Part model, mm, in its own coordinate system. A direction names the side the tool comes from. Give positions to 0.01 mm unless a question says otherwise; leave off trailing zeros. Write each loop counter-clockwise with the first axis right and the second up, starting at its lowest first coordinate (ties: lowest second). Pieces come first, ordered by that corner, then holes. Notation, with made-up numbers: M 81.5,16 L 87.5,16 A8 cw 87.5,26 Z; hole C 19.5,46.5 d1. An arc over 180 degrees is marked long. Answer as CSV lines item,"result". Start each with the question number.
Item 1: Band-saw the part on A-A, the plane z = 2.25. List the corners of the cut face in (x, y).
Item 2: 3-axis set-ups, long thin cutter, end or side, ignore diameter. For faces 4 (the cylindrical face through (0.27, 17.78, -1.4)), 5 (the flat face through (-8, 12, -2.7)), 6 (the flat face through (10.85, 12, 4)): which of +Z, -Z, +X, -X, +Y, -Y reach the whole face in a straight line?
Item 3: Band-saw the part on B-B, the plane x = 0. List the corners of the cut face in (y, z) (3 decimals).
Item 4: Band-saw the part on C-C, the plane z = -4.5. List the corners of the cut face in (x, y) (3 decimals), then the cut area to 3 significant figures.
Item 5: Wall check: L1, parallel to Y at x = 0, z = -2; L2, parallel to X at y = 4.25, z = -2.25 (1 decimal); L3, parallel to X at y = 18.25, z = -7 (3 decimals). Give the ranges that are in metal, low to high. Write a range as from..to.
Item 6: Pin check, flat tips, straight feed: pin 1 (0.6 mm diameter, centred on x = 10, y = 13, fed in from -Z); pin 2 (1 mm diameter, centred on x = 2, y = 18, fed in from +Z); pin 3 (1.8 mm diameter, centred on x = 4.5, y = 8, fed in from -Z); pin 4 (2 mm diameter, centred on x = 0, y = 19, fed in from +Z). Stop position of each tip, or through.
Item 7: Two-plate mould, pull along X, no slides. Class faces 1 (the flat face through (9.638, 12, -2)), 2 (the flat face through (-11.5, 12, -1)), 3 (the flat face through (11.5, 12, -1)): +X half, -X half, draft (parallel to the pull), parting line (faces both ways), or undercut.
from build123d import *

# Parameters (mm, degrees)
BOSS_EXTRUDE1_DEPTH         = 25
M3_TAPPED_HOLE1_D           = 2.5
M3_TAPPED_HOLE1_CSINK_D     = 3.05
M3_TAPPED_HOLE1_CSINK_ANGLE = 90


with BuildPart() as part:
    # Sketch1 → Boss-Extrude1 (new body)
    with BuildSketch(Plane(origin=(0, 0, 0), x_dir=(1, 0, 0), z_dir=(0, 1, 0))):
        with BuildLine():
            Line((-11.5, 8.7), (-10.85, 8.7))
            Line((-10.85, 8.7), (-10.85, 2.7))
            Line((-10.85, 2.7), (-9.6375, 2.7))
            Line((-9.6375, 2.7), (-9.6375, 1.775))
            ThreePointArc((-9.6375, 1.775), (-9.0125, 1.15), (-8.3875, 1.775))
            Line((-8.3875, 1.775), (-8.3875, 2.7))
            Line((-8.3875, 2.7), (-7.175, 2.7))
            Line((-7.175, 2.7), (-7.175, 8.7))
            Line((-7.175, 8.7), (-6.675, 8.7))
            Line((-6.675, 8.7), (-6.675, 1))
            Line((-6.675, 1), (-3, 1))
            Line((-3, 1), (-3, 8.7))
            Line((-3, 8.7), (-2.5, 8.7))
            Line((-2.5, 8.7), (-2.5, 2.5))
            Line((-2.5, 2.5), (2.5, 2.5))
            Line((2.5, 2.5), (2.5, 8.7))
            Line((2.5, 8.7), (3, 8.7))
            Line((3, 8.7), (3, 1))
            Line((3, 1), (6.675, 1))
            Line((6.675, 1), (6.675, 8.7))
            Line((6.675, 8.7), (7.175, 8.7))
            Line((7.175, 8.7), (7.175, 2.7))
            Line((7.175, 2.7), (8.3875, 2.7))
            Line((8.3875, 2.7), (8.3875, 1.775))
            ThreePointArc((8.3875, 1.775), (9.0125, 1.15), (9.6375, 1.775))
            Line((9.6375, 1.775), (9.6375, 2.7))
            Line((9.6375, 2.7), (10.85, 2.7))
            Line((10.85, 2.7), (10.85, 8.7))
            Line((10.85, 8.7), (11.5, 8.7))
            Line((11.5, 8.7), (11.5, -7))
            Line((11.5, -7), (10.85, -7))
            Line((10.85, -7), (10.85, 0))
            Line((10.85, 0), (-10.85, 0))
            Line((-10.85, 0), (-10.85, -7))
            Line((-10.85, -7), (-11.5, -7))
            Line((-11.5, -7), (-11.5, 8.7))
        make_face()
    extrude(amount=BOSS_EXTRUDE1_DEPTH)

    # M3 Tapped Hole1 (through all)
    with Locations(Plane.XY):
        with Locations((0, 19)):
            CounterSinkHole(M3_TAPPED_HOLE1_D / 2, M3_TAPPED_HOLE1_CSINK_D / 2, counter_sink_angle=M3_TAPPED_HOLE1_CSINK_ANGLE)


solid = part.part
Output:
1,outline,"M -11.5,0 L -10.85,0 L -10.85,25 L -11.5,25 Z; M 10.85,0 L 11.5,0 L 11.5,25 L 10.85,25 Z"
2,face 4,"+Z, -Z"
2,face 5,"-Z, +Y, -Y"
2,face 6,"+Z, +Y, -Y"
3,outline,"M 0,-2.5 L 17.75,-2.5 L 17.75,-0.275 L 17.475,0 L 0,0 Z; M 20.25,-2.5 L 25,-2.5 L 25,0 L 20.525,0 L 20.25,-0.275 Z"
4,outline,"M -11.5,0 L -10.85,0 L -10.85,25 L -11.5,25 Z; M -7.175,0 L -6.675,0 L -6.675,25 L -7.175,25 Z; M -3,0 L -2.5,0 L -2.5,25 L -3,25 Z; M 2.5,0 L 3,0 L 3,25 L 2.5,25 Z; M 6.675,0 L 7.175,0 L 7.175,25 L 6.675,25 Z; M 10.85,0 L 11.5,0 L 11.5,25 L 10.85,25 Z"
4,area,"82.5 mm²"
5,L1,"0..17.75, 20.25..25"
5,L2,"-11.5..-9.6, -8.4..-6.7, -3..3, 6.7..8.4, 9.6..11.5"
5,L3,"-11.5..-10.85, -7.175..-6.675, -3..-2.5, 2.5..3, 6.675..7.175, 10.85..11.5"
6,pin 1,"z = -2.7"
6,pin 2,"z = 0"
6,pin 3,"z = -1"
6,pin 4,"through"
7,face 1,"undercut"
7,face 2,"-X half"
7,face 3,"+X half"
